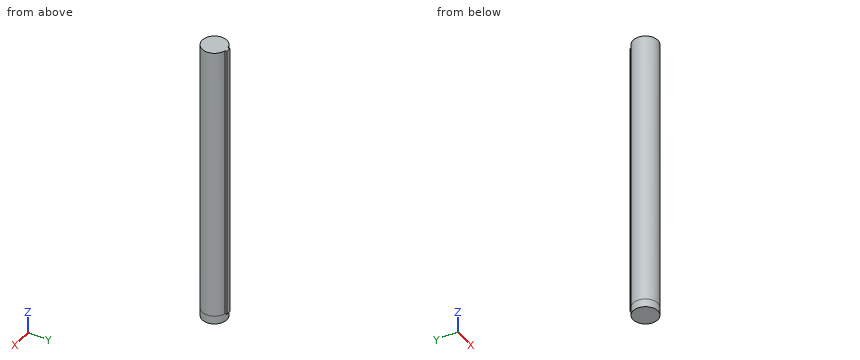
Solid Edge part; units mm, degrees
sketch "Sketch1" plane through (0, 0, 0) normal (0, 0, 1) x (1, 0, 0)
  line L0 (-1.5, 8.5) -> (1.5, 8.5)
  line L1 (-1.5, 7.3485) -> (-1.5, 8.5)
  line L2 (-1.5, 7.3485) -> (-1.5, 8.5) construction
  line L3 (1.5, 8.5) -> (1.5, 7.3485)
  arc A0 (1.5, 7.3485) -> (-1.5, 7.3485) centre (0, 0) cw
  dimension "D1" = 1.5
  dimension "D2" = 1.5
extrude "Protrusion1" add sketch "Sketch1" along normal blind 170
sketch "Sketch2" plane through (0, 0.5, 0) normal (0, 0, -1) x (0, 1, 0)
  circle A0 centre (-0.5, 0) radius 7.5
extrude "ExtrudedProtrusion_2" add sketch "Sketch2" along normal blind 5
Verification items for the finished model (mm, model axes). Coordinates: 2 decimals unless noted, no trailing zeros. Order: outer loops, then holes, each group sorted by start corner. A loop starts at its lowest first (then second) coordinate and runs counter-clockwise, first axis right, second up. Notation, with made-up numbers: (53, 8) -> (59, 8) arc R19 cw to (59, 38) -> close; hole circle Ø4 at (64, 79.5). An arc over 180 degrees is marked (long way). Answer as CSV lines item,"result". Start each with the question number.
1) Cross-section at B-B, the plane x = -4. Record the boundary of the cut face in (y, z), then the cut area to 3 significant figures.
2) Gauge pin test, flat ends, axial feed: pin 1 Ø2 at (x, z) = (6, 16.5) entering from +Y; pin 2 Ø0.9 at (y, z) = (8, 73) entering from +X. Record the tip position at first contact, or that the pin passes through.
3) Cross-section at A-A, the plane z = 125. Record the boundary of the cut face in (x, y), then the cut area to 3 significant figures.
4) Material ranges on L1, parallel to Y at x = -0.25, z = 87; L2, parallel to X at y = 7.75, z = 32.5; L3, parallel to Y at x = -4.25, z = 151.5, recorded low to high. Write a range as [from, to].
Conclusion:
1,outline,"(-6.34, -5) -> (6.34, -5) -> (6.34, 170) -> (-6.34, 170) -> close"
1,area,"2,220 mm²"
2,pin 1,"stops at y = 5.59"
2,pin 2,"stops at x = 1.5"
3,outline,"(-1.5, 7.35) arc R7.5 ccw (long way) to (1.5, 7.35) -> (1.5, 8.5) -> (-1.5, 8.5) -> close"
3,area,"180 mm²"
4,L1,"y = [-7.5, 8.5]"
4,L2,"x = [-1.5, 1.5]"
4,L3,"y = [-6.18, 6.18]"
